Read the model definition and answer for the solid it produces. Units are mm, in the model's axes. Face numbers are marked on the shaded views. Coordinates: 2 decimals unless noted, no trailing zeros. Order: outer loops, then holes, each group sorted by start corner. A loop starts at its lowest first (then second) coordinate and runs counter-clockwise, first axis right, second up. Notation, with made-up numbers: (87, 62.25) -> (141, 62.25) arc R23 cw to (141, 95.25) -> close; hole circle Ø4 at (70.25, -39.75). An arc over 180 degrees is marked (long way). Answer as a JSON object with one key per item and string values. Group by question number.
1) Determine the mould class of the marked faces 1, 2, 3 and 4 for opening direction Y: released by +Y, released by -Y, zero draft, split by the parting line, or undercut.
2) Given pin 1 (1.9 mm diameter, centred on y = -104, z = 2.5, fed in from +X); pin 2 (3 mm diameter, centred on y = -61.5, z = 5.5, fed in from +X); pin 3 (5 mm diameter, centred on x = 14.5, z = 3.5, fed in from +Y), each flat-ended and moving along its own axis, determine where each tip first touches the part or whether it passes through.
3) Section A-A on x = 10.5 is taken. Determine the outline of the cut face in (y, z).
4) Consider L1, parallel to X at y = -206.25, z = 5; L2, parallel to Y at x = 1, z = 8.75; L3, parallel to Z at x = -15, y = -204.75. Determine where each line is inside the solid, lowest interval first.
Autodesk Inventor part; units mm, degrees
ref_plane "YZ Plane" through (0, 0, 0) normal (1, 0, 0) x (0, 1, 0)
ref_plane "XZ Plane" through (0, 0, 0) normal (0, 1, 0) x (-1, 0, 0)
ref_plane "XY Plane" through (0, 0, 0) normal (0, 0, 1) x (1, 0, 0)
sketch "Skizze1" plane through (0, 0, 0) normal (0, 0, 1) x (1, 0, 0)
  line L0 (0, 42) -> (0, -252)
  line L1 (-28, 0) -> (28, 0)
  line L2 (20, 0) -> (-20, 0)
  line L3 (-20, 0) -> (-20, -210)
  line L4 (-20, -210) -> (20, -210)
  line L5 (20, -210) -> (20, 0)
  point P0 (0, 0)
  point P1 (0, -210)
  dimension "d0" = 210
  dimension "d1" = 40
extrude "Extrusion1" add sketch "Skizze1" along normal blind 10
sketch "Skizze2" plane through (0, 0, 10) normal (0, 0, 1) x (1, 0, 0)
  line L0 (20, 0) -> (20, -210)
  line L1 (-20, 0) -> (20, 0)
  line L2 (20, -8.9) -> (1, -8.9)
  line L3 (-2, -11.9) -> (-2, -18.1)
  line L4 (1, -21.1) -> (20, -21.1)
  line L5 (20, -21.1) -> (20, -8.9)
  arc A0 (1, -8.9) -> (-2, -11.9) centre (1, -11.9) ccw
  arc A1 (-2, -18.1) -> (1, -21.1) centre (1, -18.1) ccw
  line L6 (1, -12) -> (1, -18) construction
  line L7 (20, -52.4) -> (17, -52.4)
  line L8 (14, -55.4) -> (14, -64.6)
  line L9 (17, -67.6) -> (20, -67.6)
  line L10 (20, -67.6) -> (20, -52.4)
  arc A2 (17, -52.4) -> (14, -55.4) centre (17, -55.4) ccw
  arc A3 (14, -64.6) -> (17, -67.6) centre (17, -64.6) ccw
  line L11 (17, -55.5) -> (17, -64.5) construction
  line L12 (20, -98.9) -> (1, -98.9)
  line L13 (-2, -101.9) -> (-2, -108.1)
  line L14 (1, -111.1) -> (20, -111.1)
  line L15 (20, -111.1) -> (20, -98.9)
  arc A4 (1, -98.9) -> (-2, -101.9) centre (1, -101.9) ccw
  arc A5 (-2, -108.1) -> (1, -111.1) centre (1, -108.1) ccw
  line L16 (1, -102) -> (1, -108) construction
  point P0 (0, 0)
  dimension "d4" = 22
  dimension "d5" = 12.2
  dimension "d6" = 3
  dimension "d7" = 6
  dimension "d8" = 0.1
  dimension "d9" = 12
  dimension "d10" = 6
  dimension "d11" = 15.2
  dimension "d12" = 3
  dimension "d13" = 9
  dimension "d14" = 0.1
  dimension "d15" = 55.5
  dimension "d16" = 12.2
  dimension "d17" = 22
  dimension "d18" = 3
  dimension "d19" = 6
  dimension "d20" = 0.1
  dimension "d21" = 102
extrude "Extrusion2" cut sketch "Skizze2" against normal through all
sketch "Skizze3" plane through (0, 0, 0) normal (0, 0, -1) x (-1, 0, 0)
  line L0 (-20, -98.9) -> (-1, -98.9)
  line L1 (-20, 0) -> (20, 0)
  line L2 (-20, -8.9) -> (-20, 0)
  line L3 (-20, -8.9) -> (-1, -8.9)
  line L4 (-1, -21.1) -> (-20, -21.1)
  line L5 (-20, -52.4) -> (-20, -21.1)
  line L6 (-20, -52.4) -> (-17, -52.4)
  line L7 (-17, -67.6) -> (-20, -67.6)
  line L8 (-20, -98.9) -> (-20, -67.6)
  line L9 (-20, -49.4) -> (-4, -21.1)
  line L10 (-4, -8.9) -> (-4, 0)
  line L11 (-20, -70.6) -> (-4, -98.9)
  point P0 (0, 0)
  dimension "d24" = 3
  dimension "d25" = 3
  dimension "d26" = 16
  dimension "d27" = 3
  dimension "d28" = 3
extrude "Extrusion3" cut sketch "Skizze3" against normal through all
sketch "Skizze4" plane through (-20, -210, 0) normal (0, -1, 0) x (1, 0, 0)
  line L0 (0, 0) -> (40, 0)
  line L1 (40, 0) -> (40, 10)
  point P0 (20, 0)
  point P1 (5, 5)
  point P2 (35, 5)
  dimension "d31" = 30
  dimension "d32" = 5
  dimension "d33" = 5
  dimension "d34" = 5
hole "Bohrung1" at (-15, -210, 5) at (15, -210, 5) direction (0, 1, 0) diameter 4.134 depth 15 tip angle 118
equation "\"d16\" = d5"
equation "\"d17\" = d4"
equation "\"d18\" = d6"
equation "\"d27\" = d25"
equation "\"d28\" = d24"
properties part number "Olfactometer_Holder" material "Stainless Steel"
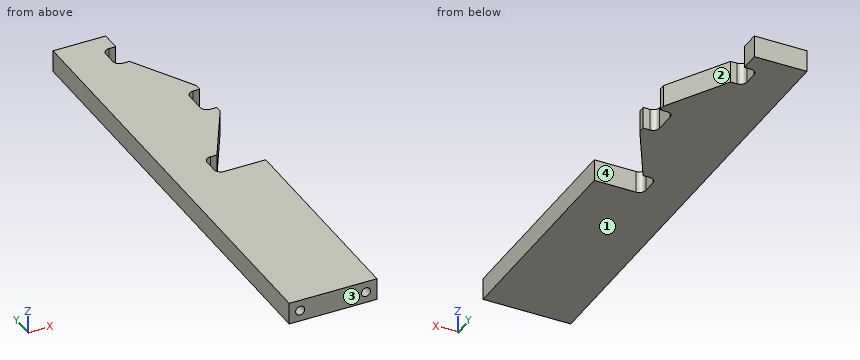
Worked answers:
{
 "1": {"face 1": "zero draft", "face 2": "released by +Y", "face 3": "released by -Y", "face 4": "undercut"},
 "2": {"pin 1": "stops at x = -2", "pin 2": "stops at x = 14", "pin 3": "stops at y = -35.25"},
 "3": {"outline": "(-210, 0) -> (-111.1, 0) -> (-111.1, 10) -> (-210, 10) -> close; (-87.4, 0) -> (-32.6, 0) -> (-32.6, 10) -> (-87.4, 10) -> close"},
 "4": {"L1": "x = -20 to -17.07, -12.93 to 12.93, 17.07 to 20", "L2": "y = -210 to -111.1, -98.9 to -21.1, -8.9 to 0", "L3": "z = 0 to 2.93, 7.07 to 10"}
}
